The listing builds one solid part. Answer for the finished solid, in the listing's coordinates (mm). Face numbers are marked on the shaded views. A direction names the side the tool comes from. Coordinates: 2 decimals unless noted, no trailing zeros. Order: outer loops, then holes, each group sorted by start corner. A loop starts at its lowest first (then second) coordinate and runs counter-clockwise, first axis right, second up.
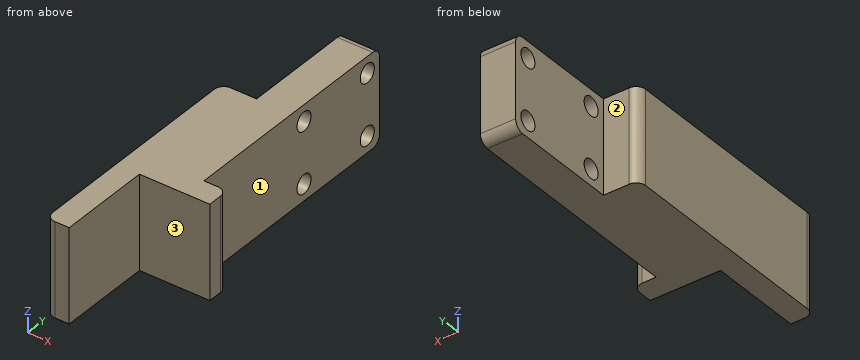
Autodesk Inventor part; units mm, degrees
ref_plane "YZ Plane" through (0, 0, 0) normal (1, 0, 0) x (0, 1, 0)
ref_plane "XZ Plane" through (0, 0, 0) normal (0, 1, 0) x (-1, 0, 0)
ref_plane "XY Plane" through (0, 0, 0) normal (0, 0, 1) x (1, 0, 0)
sketch "Sketch1" plane through (0, 0, 0) normal (0, 0, 1) x (1, 0, 0)
  line L0 (0, -20) -> (0, 0)
  line L1 (0, 0) -> (15, 0)
  line L2 (-5, -20) -> (-5, 5)
  line L3 (-5, 5) -> (15, 5)
  line L4 (0, -20) -> (-5, -20)
  line L5 (15, 5) -> (15, 0)
  dimension "d0" = 15
  dimension "d1" = 20
  dimension "d2" = 5
extrude "Extrusion1" add sketch "Sketch1" along normal blind 20
sketch "Sketch2" plane through (-5, 5, 0) normal (0, 1, 0) x (1, 0, 0)
  line L0 (0, 0) -> (20, 0)
  line L1 (20, -20) -> (0, -20)
  line L2 (0, 0) -> (0, -20)
  line L3 (15, 0) -> (15, -20)
  line L4 (0, 0) -> (15, 0)
  line L5 (20, 0) -> (5, 0)
  line L6 (15, -20) -> (0, -20)
  line L7 (0, 0) -> (0, -20)
  dimension "d7" = 0
  dimension "d8" = 15
extrude "Extrusion2" add sketch "Sketch2" along normal blind 25
sketch "Sketch3" plane through (-5, 30, 0) normal (0, 1, 0) x (1, 0, 0)
  line L0 (15, 0) -> (15, -20)
  line L1 (15, 0) -> (7.5, 0)
  line L2 (7.5, 0) -> (7.5, -20)
  line L3 (7.5, -20) -> (15, -20)
  line L4 (15, -20) -> (15, 0)
  point P0 (5, 0)
  dimension "d11" = 7.5
  dimension "d12" = 20
extrude "Extrusion3" add sketch "Sketch3" along normal blind 25
sketch "Sketch4" plane through (2.5, 30, 0) normal (-1, 0, 0) x (0, 0, 1)
  line L0 (0, 25) -> (20, 25)
  line L1 (10, 25) -> (10, 0)
  line L2 (20, 0) -> (0, 0)
  line L3 (0, 0) -> (0, 25)
  line L4 (0, 12.5) -> (20, 12.5)
  line L5 (20, -25) -> (20, 25)
  circle A0 centre (3.5, 21.5) radius 2
  circle A1 centre (16.5, 21.5) radius 2
  circle A2 centre (3.5, 3.5) radius 2
  circle A3 centre (16.5, 3.5) radius 2
  point P0 (0, -30)
  dimension "d15" = 4
  dimension "d16" = 3.5
  dimension "d17" = 3.5
hole "Hole1" at (2.5, 51.5, 3.5) at (2.5, 51.5, 16.5) at (2.5, 33.5, 16.5) at (2.5, 33.5, 3.5) direction (1, 0, 0) diameter 4 end through all
fillet "Fillet1" radius 2 5 edges at (-5, 30, 10) (6.25, 55, 0) (6.25, 55, 20) (15, 5, 10) (-5, -20, 10)
properties part number "Esteira - Carro"
(1) For the marked faces 1, 2 and 3, determine the directions among +Z, -Z, +X, -X, +Y, -Y from which every point of the face is accessible in a straight line to the end or side of a thin tool.
(2) Find section A-A (x = 6.75). Write down the section's boundary in (y, z), and give its area (3 significant figures).
(3) Find section C-C (z = 16.5). Write down the section's boundary in (x, y).
(4) Each of these flat-tipped pins is pushed along its axis until it touches: pin 1 Ø1.6 at (x, z) = (1, 8) entering from +Y; pin 2 Ø6 at (y, z) = (46.5, 14) entering from +X; pin 3 Ø6 at (x, z) = (7.5, 16.5) entering from -Y; pin 4 Ø3.5 at (y, z) = (33.5, 16.5) entering from -X. Where does it stop, or does it pass through?
(5) Find section B-B (y = 33.5). Write down the section's boundary in (x, z), and give its area (3 significant figures).
(6) Find section D-D (z = 10.5). Write down the section's boundary in (x, y), and give its area (3 significant figures).
(7) Consider line 1 (Z direction, x = 6.75, y = 33.5); line 2 (Y direction, x = 6, z = 16.5); line 3 (Y direction, x = 2.75, z = 4). Determine where each line is inside the solid, lowest interval first.
Findings below:
1. face 1: +Z, -Z, +X, +Y
1. face 2: +Z, -Z, -X, +Y
1. face 3: +Z, -Z, +X, -Y
2. outline: (0, 0) - (53, 0) arc R2 ccw to (55, 2) - (55, 18) arc R2 ccw to (53, 20) - (0, 20) - close; hole circle Ø4 at (33.5, 3.5); hole circle Ø4 at (33.5, 16.5); hole circle Ø4 at (51.5, 3.5); hole circle Ø4 at (51.5, 16.5)
2. area: 1,050 mm2
3. outline: (-5, -18) arc R2 ccw to (-3, -20) - (0, -20) - (0, 0) - (15, 0) - (15, 3) arc R2 ccw to (13, 5) - (10, 5) - (10, 31.5) - (2.5, 31.5) - (2.5, 30) - (-3, 30) arc R2 ccw to (-5, 28) - close; (2.5, 35.5) - (10, 35.5) - (10, 49.5) - (2.5, 49.5) - close; (2.5, 53.5) - (10, 53.5) - (10, 55) - (2.5, 55) - close
4. pin 1: stops at y = 30
4. pin 2: stops at x = 10
4. pin 3: stops at y = 0
4. pin 4: passes through
5. outline: (2.5, 0) - (10, 0) - (10, 1.5) - (2.5, 1.5) - close; (2.5, 5.5) - (10, 5.5) - (10, 14.5) - (2.5, 14.5) - close; (2.5, 18.5) - (10, 18.5) - (10, 20) - (2.5, 20) - close
5. area: 90.0 mm2
6. outline: (-5, -18) arc R2 ccw to (-3, -20) - (0, -20) - (0, 0) - (15, 0) - (15, 3) arc R2 ccw to (13, 5) - (10, 5) - (10, 55) - (2.5, 55) - (2.5, 30) - (-3, 30) arc R2 ccw to (-5, 28) - close
6. area: 760 mm2
7. line 1: z = 0 to 1.5, 5.5 to 14.5, 18.5 to 20
7. line 2: y = 0 to 31.5, 35.5 to 49.5, 53.5 to 55
7. line 3: y = 0 to 31.56, 35.44 to 49.56, 53.44 to 55
